Geometry: final body of the model. Coordinates: model frame, mm. Face numbers are marked on the shaded views. A direction names the side the tool comes from. Round coordinates to 2 decimals unless told otherwise and drop trailing zeros. Write each loop counter-clockwise with the first axis right and the second up, starting at its lowest first coordinate (ties: lowest second). Pieces come first, ordered by that corner, then holes. Notation, with made-up numbers: M 24,8 L 65,8 A15 cw 65,31 Z; hole C -10.5,17 d11. An arc over 180 degrees is marked long. Answer as CSV lines item,"result". Start each with the question number.
Q1. Section query A-A on y = 0. Output: boundary loops of the cut face in (x, z), and give its area (3 significant figures).
Q2. Ray query, probe 1 along Y at (x, z) = (-20, 1.3); probe 2 along Y at (x, z) = (10.5, -1.3); probe 3 along X at (y, z) = (0, -0.5). Return the intervals inside material, ascending.
Q3. Reachability of the marked faces 1 and 2 from +Z, -Z, +X, -X, +Y, -Y: full face, straight path, thin tool, end or side. Return the list, or none.
Q4. Mould query, pull axis Y, two halves, no side actions, for the marked faces 3, 4 and 5. Classes: pulls with the +Y half, pulls with the -Y half, needs draft (parallel to the pull), parting line crosses it, or undercut.
Q5. Section query D-D on y = 10. Output: boundary loops of the cut face in (x, z), and give its area (3 significant figures).
Q6. First-contact query: pin 1 (9 mm diameter, centred on x = -10, y = -2.5, fed in from -Z); pin 2 (1.6 mm diameter, centred on x = -10.5, y = 12.5, fed in from -Z); pin 3 (2 mm diameter, centred on x = 1, y = -7.5, fed in from -Z); pin 4 (1.2 mm diameter, centred on x = -10.5, y = 12.5, fed in from +Z). Flat tips, straight axial feed; report the tip coordinate or a pass-through.
Q7. Section query B-B on x = -21. Output: boundary loops of the cut face in (y, z).
Q8. Section query C-C on z = 1.5. Output: boundary loops of the cut face in (x, y), and give its area (3 significant figures).
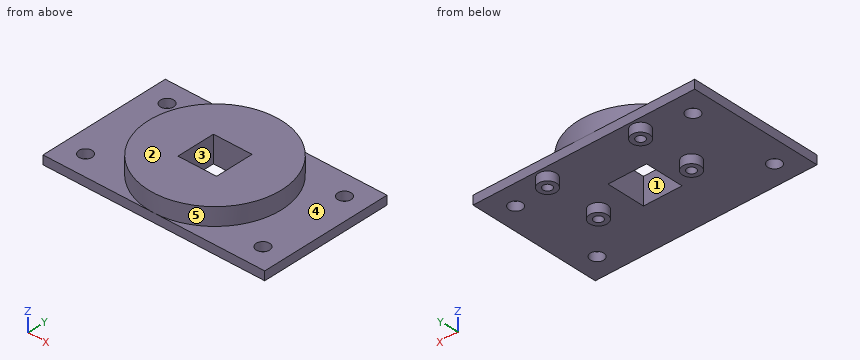
```python
from build123d import *

# Parameters (mm, degrees)
SKETCH_W        = 50
SKETCH_H        = 30
SKETCH_R        = 1.5
PAD_DEPTH       = 2
SKETCH001_R     = 15
PAD001_DEPTH    = 4
SKETCH002_W     = 8.7
SKETCH002_H     = 8.7
POCKET_DEPTH    = 7
SKETCH003_R     = 2
PAD002_DEPTH    = 2
SKETCH004_R     = 1
POCKET001_DEPTH = 3


with BuildPart() as part:
    # Sketch → Pad (new body)
    with BuildSketch(Plane.XY):
        Rectangle(SKETCH_W, SKETCH_H)
        with Locations((-20, 10)):
            Circle(SKETCH_R, mode=Mode.SUBTRACT)
        with Locations((-20, -10)):
            Circle(SKETCH_R, mode=Mode.SUBTRACT)
        with Locations((20, -10)):
            Circle(SKETCH_R, mode=Mode.SUBTRACT)
        with Locations((20, 10)):
            Circle(SKETCH_R, mode=Mode.SUBTRACT)
    extrude(amount=PAD_DEPTH)

    # Sketch001 → Pad001 (new body)
    with BuildSketch(Plane.XY.offset(2)):
        Circle(SKETCH001_R)
    extrude(amount=PAD001_DEPTH)

    # Sketch002 → Pocket (cut)
    with BuildSketch(Plane.XY.offset(6)):
        Rectangle(SKETCH002_W, SKETCH002_H)
    extrude(amount=-POCKET_DEPTH, mode=Mode.SUBTRACT)

    # Sketch003 → Pad002 (new body)
    with BuildSketch(Plane(origin=(0, 0, 0), x_dir=(1, 0, 0), z_dir=(0, 0, -1))):
        with Locations((-10.5, 0)):
            Circle(SKETCH003_R)
        with Locations((10.5, -12.5)):
            Circle(SKETCH003_R)
        with Locations((-10.5, -12.5)):
            Circle(SKETCH003_R)
        with Locations((10.5, 0)):
            Circle(SKETCH003_R)
    extrude(amount=PAD002_DEPTH)

    # Sketch004 → Pocket001 (cut)
    with BuildSketch(Plane(origin=(0, 0, -2), x_dir=(1, 0, 0), z_dir=(0, 0, -1))):
        with Locations((-10.5, 0)):
            Circle(SKETCH004_R)
        with Locations((10.5, 0)):
            Circle(SKETCH004_R)
        with Locations((10.5, -12.5)):
            Circle(SKETCH004_R)
        with Locations((-10.5, -12.5)):
            Circle(SKETCH004_R)
    extrude(amount=-POCKET001_DEPTH, mode=Mode.SUBTRACT)


solid = part.part
```
Entries:
1,outline,"M -25,0 L -12.5,0 L -12.5,-2 L -11.5,-2 L -11.5,1 L -9.5,1 L -9.5,-2 L -8.5,-2 L -8.5,0 L -4.35,0 L -4.35,6 L -15,6 L -15,2 L -25,2 Z; M 4.35,0 L 8.5,0 L 8.5,-2 L 9.5,-2 L 9.5,1 L 11.5,1 L 11.5,-2 L 12.5,-2 L 12.5,0 L 25,0 L 25,2 L 15,2 L 15,6 L 4.35,6 Z"
1,area,"172 mm^2"
2,probe 1,"y = -15 to -11.5, -8.5 to 8.5, 11.5 to 15"
2,probe 2,"y = -2 to -1, 1 to 2, 10.5 to 11.5, 13.5 to 14.5"
2,probe 3,"x = -12.5 to -11.5, -9.5 to -8.5, 8.5 to 9.5, 11.5 to 12.5"
3,face 1,"+Z, -Z"
3,face 2,"+Z, +X, -X, +Y, -Y"
4,face 3,"undercut"
4,face 4,"needs draft"
4,face 5,"parting line crosses it"
5,outline,"M -25,0 L -21.5,0 L -21.5,2 L -25,2 Z; M -18.5,0 L 18.5,0 L 18.5,2 L 11.18,2 L 11.18,6 L -11.18,6 L -11.18,2 L -18.5,2 Z; M 21.5,0 L 25,0 L 25,2 L 21.5,2 Z"
5,area,"177 mm^2"
6,pin 1,"stops at z = -2"
6,pin 2,"stops at z = 1"
6,pin 3,"stops at z = 0"
6,pin 4,"stops at z = 2"
7,outline,"M -15,0 L -11.12,0 L -11.12,2 L -15,2 Z; M -8.88,0 L 8.88,0 L 8.88,2 L -8.88,2 Z; M 11.12,0 L 15,0 L 15,2 L 11.12,2 Z"
8,outline,"M -25,-15 L 25,-15 L 25,15 L -25,15 Z; hole C -20,-10 d3; hole C -20,10 d3; hole M -4.35,-4.35 L 4.35,-4.35 L 4.35,4.35 L -4.35,4.35 Z; hole C 20,-10 d3; hole C 20,10 d3"
8,area,"1,400 mm^2"
